```python
from build123d import *

# Parameters (mm, degrees)
F0_W     = 50
F0_H     = 40
F1_DEPTH = 20
F3_DEPTH = 20
F5_DEPTH = 20


with BuildPart() as f1:
    # F0 (on Top) → F1 (new body)
    with BuildSketch(Plane.XY):
        with Locations((25, 20)):
            Rectangle(F0_W, F0_H)
    extrude(amount=F1_DEPTH)

    # F2 (on face) → F3 (join)
    with BuildSketch(Plane.XY.offset(20)):
        with BuildLine():
            Line((0, 40), (0, 0))
            ThreePointArc((0, 0), (14.142136, 5.857864), (20, 20))
            Line((20, 20), (20, 40))
            Line((20, 40), (0, 40))
        make_face()
    extrude(amount=F3_DEPTH)

    # F4 (on face) → F5 (join)
    with BuildSketch(Plane(origin=(0, 40, 0), x_dir=(-1, 0, 0), z_dir=(0, 1, 0))):
        Polygon((-20, 20), (-20, 40), (-50, 20), align=None)
    extrude(amount=-F5_DEPTH)


solid = f1.part
```
For this review, take the finished solid that the model builds, in its own axes (mm). A direction names the side the tool comes from. Coordinates: 2 decimals unless noted, no trailing zeros. Write each loop counter-clockwise with the first axis right and the second up, starting at its lowest first coordinate (ties: lowest second). Pieces come first, ordered by that corner, then holes.
(1) The part is to be moulded in two halves that separate along X. For faces 3 (the face through (35, 30, 30)), 4 (the face through (0, 20, 20)), 5 (the face through (30, 10, 20)), say which applies: +X half, -X half, draft (parallel to the pull), parting line (faces both ways), or undercut.
(2) Tool access review of faces 1 (the face through (25, 0, 10)), 2 (the face through (13.986, 5.703, 29.86)): name each direction out of +Z, -Z, +X, -X, +Y, -Y from which nothing blocks a thin tool from reaching the whole face with its end or side.
(3) For pin 1 Ø10 at (x, y) = (39, 22) entering from +Z; pin 2 Ø10 at (x, z) = (37.5, 32) entering from -Y, all flat-tipped, find the tip position at first contact; note any pin that passes through.
(4) Add section B-B on z = 27.5. Give the boundary of the cut face in (x, y).
(5) Add section D-D on x = 41. Give the boundary of the cut face in (y, z), then the cut area to 3 significant figures.
(6) Add section A-A on x = 32. Give the boundary of the cut face in (y, z).
(7) Add section C-C on y = 23. Give the boundary of the cut face in (x, z).
(8) Wall thickness on probe 1 along Y at (x, z) = (23.5, 21); probe 2 along Z at (x, y) = (45, 16.5); probe 3 along Z at (x, y) = (24.5, 22): over which ranges is each line inside the solid? List them lowest first.
Answer sheet:
1. face 3: +X half
1. face 4: -X half
1. face 5: draft
2. face 1: +Z, -Z, +X, -X, -Y
2. face 2: +Z, +X, -Y
3. pin 1: stops at z = 30.67
3. pin 2: stops at y = 20
4. outline: (0, 0) arc R20 ccw to (20, 20) - (38.75, 20) - (38.75, 40) - (0, 40) - close
5. outline: (0, 0) - (40, 0) - (40, 26) - (20, 26) - (20, 20) - (0, 20) - close
5. area: 920 mm2
6. outline: (0, 0) - (40, 0) - (40, 32) - (20, 32) - (20, 20) - (0, 20) - close
7. outline: (0, 0) - (50, 0) - (50, 20) - (20, 40) - (0, 40) - close
8. probe 1: y = 20 to 40
8. probe 2: z = 0 to 20
8. probe 3: z = 0 to 37
